Autodesk Inventor part; units mm, degrees
ref_plane "YZ Plane" through (0, 0, 0) normal (1, 0, 0) x (0, 1, 0)
ref_plane "XZ Plane" through (0, 0, 0) normal (0, 1, 0) x (-1, 0, 0)
ref_plane "XY Plane" through (0, 0, 0) normal (0, 0, 1) x (1, 0, 0)
sketch "Skizze1" plane through (0, 0, 0) normal (0, 0, 1) x (1, 0, 0)
  line L0 (0, 0) -> (6.75, 0)
  line L1 (6.75, 0) -> (6.75, 4.9)
  line L2 (6.75, 4.9) -> (3.75, 4.9)
  line L3 (3.75, 4.9) -> (3.75, 10.2)
  line L4 (3.75, 10.2) -> (18.25, 10.2)
  line L5 (18.25, 10.2) -> (18.25, 4.9)
  line L6 (18.25, 4.9) -> (15.25, 4.9)
  line L7 (15.25, 4.9) -> (15.25, 0)
  line L8 (15.25, 0) -> (22, 0)
  line L9 (22, 0) -> (22, 80.2)
  line L10 (0, 0) -> (0, 68.2123)
  line L11 (22, 80.2) -> (22, 98.8308) construction
  line L12 (22, 80.2) -> (17.076, 79.3318)
  line L13 (17.076, 79.3318) -> (15.3395, 89.1798)
  arc A0 (22, 90.2123) -> (15.3395, 89.1798) centre (22, 68.2123) ccw construction
  arc A1 (15.3395, 89.1798) -> (0, 68.2123) centre (22, 68.2123) ccw
  dimension "d0" = 14.5
  dimension "d1" = 5.3
  dimension "d2" = 4.9
  dimension "d3" = 22
  dimension "d4" = 8.5
  dimension "d5" = 5
  dimension "d6" = 10
  dimension "d21" = 70
  dimension "d22" = 80
extrude "Extrusion1" add sketch "Skizze1" along normal blind 22
sketch "Skizze2" plane through (22, 0, 0) normal (1, 0, 0) x (0, 0, -1)
  circle A0 centre (-11, 7.5) radius 2
  line L0 (0, 0) -> (-22, 0)
  line L1 (0, 0) -> (0, 80.2)
  point P0 (0, 65.2)
  dimension "d10" = 4
  dimension "d11" = 7.5
  dimension "d12" = 11
extrude "Extrusion2" cut sketch "Skizze2" against normal blind 22
chamfer "Fasen1" distance 1 angle 45 18 edges at (3.75, 7.55, 22) (11, 10.2, 22) (18.25, 7.55, 22) (16.75, 4.9, 22) (5.25, 4.9, 22) (6.75, 2.45, 22) (15.25, 2.45, 22) (18.25, 7.55, 0) (15.25, 2.45, 0) (16.75, 4.9, 0) (11, 10.2, 0) (3.75, 7.55, 0) (5.25, 4.9, 0) (6.75, 2.45, 0) (6.75, 4.9, 11) (15.25, 4.9, 11) (6.75, 0, 11) (15.25, 0, 11)
sketch "Skizze4" plane through (17.076, 79.3318, 22) normal (-0.1736482, 0.9848078, 0) x (0.9848078, 0.1736482, 0)
  line L0 (-18.7474, 0) -> (0, 0)
  line L1 (5, 22) -> (5, 0)
  line L2 (0, 0) -> (5, 0)
  line L3 (5, 0) -> (5, 3.5)
  line L4 (5, 3.5) -> (0, 3.5)
  line L5 (0, 3.5) -> (0, 0)
  line L6 (-8.9266, 22) -> (5, 22)
  line L7 (0, 22) -> (5, 22)
  line L8 (5, 22) -> (5, 18.5)
  line L9 (5, 18.5) -> (0, 18.5)
  line L10 (0, 18.5) -> (0, 22)
  point P0 (-30.5924, 22)
  point P1 (2.5, 18.5)
  point P2 (5, 18.5)
  point P3 (5, 0)
  dimension "d29" = 15
extrude "Extrusion4" add sketch "Skizze4" along normal blind 10
properties part number "Gripper_V2_10deg"
Verification items for the finished model (mm, model axes). A direction names the side the tool comes from. Coordinates: 2 decimals unless noted, no trailing zeros. Order: outer loops, then holes, each group sorted by start corner. A loop starts at its lowest first (then second) coordinate and runs counter-clockwise, first axis right, second up. Notation, with made-up numbers: (57.25, -18) -> (92.25, -18) arc R5 ccw to (92.25, -11) -> close; hole circle Ø6 at (57, -13.75). An arc over 180 degrees is marked (long way). Answer as CSV lines item,"result". Start each with the question number.
1) Release check for a two-part mould opening along Z. For faces 4 (the face through (11, 46, 0)), 5 (the face through (11, 46, 22)), 6 (the face through (19.57, 79.77, 10.9)) record: released by +Z, released by -Z, zero draft, split by the parting line, or undercut.
2) Gauge pin test, flat ends, axial feed: pin 1 Ø5 at (x, z) = (15.5, 13.5) entering from +Y; pin 2 Ø7 at (x, z) = (9.5, 8.5) entering from -Y; pin 3 Ø2 at (x, z) = (5, 8) entering from +Y; pin 4 Ø2.5 at (y, z) = (7.5, 11) entering from -X. Record the tip position at first contact, or that the pin passes through.
3) Cross-section at D-D, the plane y = 75.5. Record the boundary of the cut face in (x, z), then the cut area to 3 significant figures.
4) Cross-section at B-B, the plane z = 11.5. Record the boundary of the cut face in (x, y), then the cut area to 3 significant figures.
5) Set-up check for faces 1 (the face through (3.75, 7.5, 8.6)), 2 (the face through (21.144, 85.055, 1.726)), 3 (the face through (15.25, 2, 11)): record each of +Z, -Z, +X, -X, +Y, -Y from which the full face is reachable in a straight line by a thin tool's end or side.
6) Cross-section at C-C, the plane z = 15. Record the boundary of the cut face in (x, y).
7) Material ranges on L1, parallel to Y at x = 2.4, z = 11; L2, parallel to Y at x = 20.45, z = 11; L3, parallel to X at y = 75, z = 18.5, recorded low to high. Write a range as [from, to].
8) Cross-section at A-A, the plane y = 7.5. Record the boundary of the cut face in (x, z).
Conclusion:
1,face 4,"released by -Z"
1,face 5,"released by +Z"
1,face 6,"undercut"
2,pin 1,"stops at y = 89.18"
2,pin 2,"stops at y = 0.25"
2,pin 3,"stops at y = 83.31"
2,pin 4,"passes through"
3,outline,"(1.24, 0) -> (22, 0) -> (22, 22) -> (1.24, 22) -> close"
3,area,"457 mm²"
4,outline,"(0, 0) -> (5.75, 0) -> (6.75, 1) -> (6.75, 3.9) -> (5.75, 4.9) -> (3.75, 4.9) -> (3.75, 5.56) -> (0, 5.56) -> close; (0, 9.44) -> (3.75, 9.44) -> (3.75, 10.2) -> (18.25, 10.2) -> (18.25, 9.44) -> (22, 9.44) -> (22, 80.2) -> (17.08, 79.33) -> (15.34, 89.18) arc R22 ccw to (0, 68.21) -> close; (15.25, 1) -> (16.25, 0) -> (22, 0) -> (22, 5.56) -> (18.25, 5.56) -> (18.25, 4.9) -> (16.25, 4.9) -> (15.25, 3.9) -> close"
4,area,"1,670 mm²"
5,face 1,"+Z, -Z"
5,face 2,"+Z, -Z, +X, +Y"
5,face 3,"+Z, -Z, -Y"
6,outline,"(0, 0) -> (5.75, 0) -> (6.75, 1) -> (6.75, 3.9) -> (5.75, 4.9) -> (3.75, 4.9) -> (3.75, 10.2) -> (18.25, 10.2) -> (18.25, 4.9) -> (16.25, 4.9) -> (15.25, 3.9) -> (15.25, 1) -> (16.25, 0) -> (22, 0) -> (22, 80.2) -> (17.08, 79.33) -> (15.34, 89.18) arc R22 ccw to (0, 68.21) -> close"
7,L1,"y = [0, 5.5], [9.5, 78.2]"
7,L2,"y = [0, 5.5], [9.5, 79.93]"
7,L3,"x = [1.07, 22]"
8,outline,"(0, 0) -> (2.75, 0) -> (3.75, 1) -> (3.75, 9) -> (0, 9) -> close; (0, 13) -> (3.75, 13) -> (3.75, 21) -> (2.75, 22) -> (0, 22) -> close; (18.25, 1) -> (19.25, 0) -> (22, 0) -> (22, 9) -> (18.25, 9) -> close; (18.25, 13) -> (22, 13) -> (22, 22) -> (19.25, 22) -> (18.25, 21) -> close"
